Part model, mm, in its own coordinate system. Face numbers are marked on the shaded views. A direction names the side the tool comes from. Round coordinates to 2 decimals unless told otherwise and drop trailing zeros. Write each loop counter-clockwise with the first axis right and the second up, starting at its lowest first coordinate (ties: lowest second). Pieces come first, ordered by that corner, then holes.
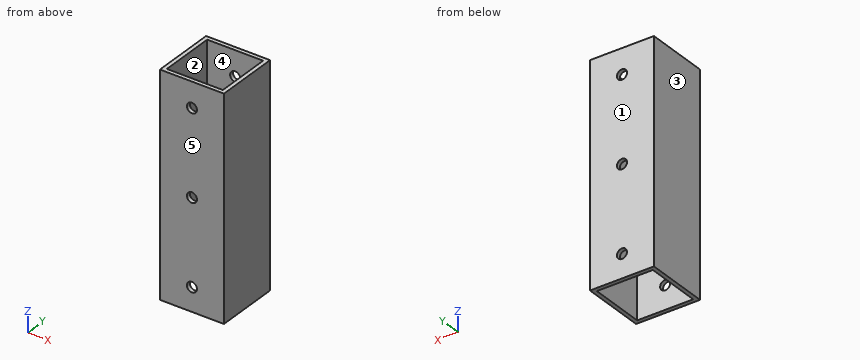
Autodesk Inventor part; units mm, degrees
ref_plane "YZ Plane" through (0, 0, 0) normal (1, 0, 0) x (0, 1, 0)
ref_plane "XZ Plane" through (0, 0, 0) normal (0, 1, 0) x (-1, 0, 0)
ref_plane "XY Plane" through (0, 0, 0) normal (0, 0, 1) x (1, 0, 0)
sketch "Sketch1" plane through (0, 0, 0) normal (0, 0, 1) x (1, 0, 0)
  line L0 (0, 0) -> (50.8, 0)
  line L1 (50.8, 0) -> (50.8, 50.8)
  line L2 (50.8, 50.8) -> (0, 50.8)
  line L3 (0, 50.8) -> (0, 0)
  line L4 (3.175, 3.175) -> (47.625, 3.175)
  line L5 (47.625, 3.175) -> (47.625, 47.625)
  line L6 (47.625, 47.625) -> (3.175, 47.625)
  line L7 (3.175, 47.625) -> (3.175, 3.175)
  dimension "d0" = 50.8
  dimension "d1" = 50.8
  dimension "d2" = 3.175
extrude "Extrusion1" add sketch "Sketch1" along normal blind 263.05
sketch "Sketch2" plane through (0, 0, 0) normal (0, -1, 0) x (1, 0, 0)
  circle A0 centre (25.4, 107.63) radius 4
  line L0 (0, 0) -> (50.8, 0)
  circle A1 centre (25.4, 175.34) radius 4
  circle A2 centre (25.4, 243.05) radius 4
  point P0 (25.4, 0)
  dimension "d5" = 8
  dimension "d6" = 107.63
  dimension "d7" = 8
  dimension "d8" = 8
  dimension "d9" = 67.71
  dimension "d10" = 67.71
extrude "Extrusion2" cut sketch "Sketch2" against normal through all
sketch "Sketch3" plane through (0, 0, 0) normal (0, -1, 0) x (1, 0, 0)
  line L0 (50.8, 0) -> (50.8, 263.05)
  line L1 (0, 0) -> (50.8, 0)
  line L2 (50.8, 0) -> (50.8, 88.9)
  line L3 (50.8, 88.9) -> (0, 88.9)
  line L4 (0, 88.9) -> (0, 0)
  dimension "d13" = 88.9
extrude "Extrusion3" cut sketch "Sketch3" against normal through all
properties part number "ST01" material "Aluminum 6061"
Q1. Mould opens along Y. For the marked faces 1, 2 and 3 say: +Y half, -Y half, draft (parallel to the pull), parting line (faces both ways), or undercut.
Values follow:
face 1: +Y half
face 2: undercut
face 3: draft
Q2. Cut at B-B on z = 175.34. Write the cut outline in (x, y) (3 decimals), plus the area to 3 significant figures.
Values follow:
outline: (0, 0) - (21.4, 0) - (21.4, 3.175) - (3.175, 3.175) - (3.175, 47.625) - (21.4, 47.625) - (21.4, 50.8) - (0, 50.8) - close; (29.4, 0) - (50.8, 0) - (50.8, 50.8) - (29.4, 50.8) - (29.4, 47.625) - (47.625, 47.625) - (47.625, 3.175) - (29.4, 3.175) - close
area: 554 mm2
Q3. Wall check: L1, parallel to Y at x = 30, z = 131.5 (3 decimals); L2, parallel to X at y = 50, z = 107. Give the ranges that are in metal, low to high.
Values follow:
L1: y = 0 to 3.175, 47.625 to 50.8
L2: x = 0 to 21.45, 29.35 to 50.8
Q4. Cut at C-C on x = 25.4. State how many separate pieces and enclosed holes the cut face has, plus the area to 3 significant figures.
Values follow:
separate pieces: 8
enclosed holes: 0
area: 953 mm2
Q5. Cut at A-A on x = 37.5. Write the cut outline in (y, z) (3 decimals), plus the area to 3 significant figures.
Values follow:
outline: (0, 88.9) - (3.175, 88.9) - (3.175, 263.05) - (0, 263.05) - close; (47.625, 88.9) - (50.8, 88.9) - (50.8, 263.05) - (47.625, 263.05) - close
area: 1,110 mm2
Q6. Drop a flat-ended pin along its axis: pin 1 (2 mm diameter, centred on y = 26.5, z = 151.5, fed in from -X). Give the stop position or say it passes through.
Values follow:
pin 1: stops at x = 0
Q7. Which spindle directions (+Z, -Z, +X, -X, +Y, -Y) get a long thin tool onto all of the face, cutting with end or side? Do the marked faces 4 and 5. Say none if no direction does.
Values follow:
face 4: +Z, -Z
face 5: +Z, -Z, +X, -X, -Y
